For this review, take the finished solid that the model builds, in its own axes (mm). A direction names the side the tool comes from. Coordinates: 2 decimals unless noted, no trailing zeros. Loops run counter-clockwise (first coordinate to the right, second up) from the corner with the lowest first, then second, coordinate; pieces in that order, holes last. Notation, with made-up numbers: (12, 9) - (38, 9) arc R34 cw to (38, 43) - close; hole circle Ø9 at (21.5, 66.25). An arc over 180 degrees is marked (long way). Answer as a JSON object with one key per item and string values. Group by question number.
Item 1: To check wall thickness, follow line 1 (Y direction, x = -9.5, z = 2.2); line 2 (X direction, y = 2, z = 0.35); line 3 (Z direction, x = -26, y = -3). State the ranges of each line that lie inside material, in increasing order.
Item 2: We need section B-B (x = 29). Give the boundary of the cut face in (y, z).
Item 3: We need section A-A (y = 0). State how many separate pieces and enclosed holes the cut face has, then the cut area to 3 significant figures.
Item 4: Mouldability with a two-part tool opening along Y and no side actions: class faces 3 (the flat face through (-50, 0, -0.625)), 4 (the cylindrical face through (-46.01, 14.79, 1.23)), 5 (the cylindrical face through (-45.281, -13.774, 1.866)) as released by +Y, released by -Y, zero draft, split by the parting line, or undercut.
Item 5: Clearance check with flat-ended pins moving along their axes: pin 1 (2 mm diameter, centred on x = 12.5, y = -5, fed in from +Z); pin 2 (6 mm diameter, centred on x = 47, y = 0, fed in from +Z) (3 decimals). State where each tip first meets the part, or that it passes through.
Item 6: Tool access review of faces 1 (the flat face through (-1, 0, 1.25)), 2 (the flat face through (-56, 0, 1)): name each direction out of +Z, -Z, +X, -X, +Y, -Y from which nothing blocks a thin tool from reaching the whole face with its end or side.
from build123d import *

# Parameters (mm, degrees)
BOSS_EXTRUDE1_DEPTH      = 2.5
SKETCH1_3_R              = 3.75
BOSS_EXTRUDE2_DEPTH      = 1.25
BOSS_EXTRUDE4_DEPTH      = 1.875
BOSS_EXTRUDE4_DEPTH_BACK = 0.625
SKETCH1_4_R              = 3.75
SKETCH1_4_R_2            = 2.5


with BuildPart() as part:
    # Sketch1 → Boss-Extrude1 (new body)
    with BuildSketch(Plane.XY):
        with BuildLine():
            ThreePointArc((-53.352941176, 6.898076983), (-55.26649875, 5.541774365), (-56, 3.313942393))
            Line((-56, 3.313942393), (-56, -3.313942393))
            ThreePointArc((-56, -3.313942393), (-55.26649875, -5.541774365), (-53.352941176, -6.898076983))
            ThreePointArc((-53.352941176, -6.898076983), (-49.636038969, -9.136038969), (-47.398076983, -12.852941176))
            ThreePointArc((-47.398076983, -12.852941176), (-46.041774365, -14.76649875), (-43.813942393, -15.5))
            Line((-43.813942393, -15.5), (0, -15.5))
            Line((0, -15.5), (43.813942393, -15.5))
            ThreePointArc((43.813942393, -15.5), (46.041774365, -14.76649875), (47.398076983, -12.852941176))
            ThreePointArc((47.398076983, -12.852941176), (49.636038969, -9.136038969), (53.352941176, -6.898076983))
            ThreePointArc((53.352941176, -6.898076983), (55.26649875, -5.541774365), (56, -3.313942393))
            Line((56, -3.313942393), (56, 3.313942393))
            ThreePointArc((56, 3.313942393), (55.26649875, 5.541774365), (53.352941176, 6.898076983))
            ThreePointArc((53.352941176, 6.898076983), (49.636038969, 9.136038969), (47.398076983, 12.852941176))
            ThreePointArc((47.398076983, 12.852941176), (46.041774365, 14.76649875), (43.813942393, 15.5))
            Line((43.813942393, 15.5), (0, 15.5))
            Line((0, 15.5), (-43.813942393, 15.5))
            ThreePointArc((-43.813942393, 15.5), (-46.041774365, 14.76649875), (-47.398076983, 12.852941176))
            ThreePointArc((-47.398076983, 12.852941176), (-49.636038969, 9.136038969), (-53.352941176, 6.898076983))
        make_face()
        with BuildLine():
            Line((43.813942393, -14.25), (0, -14.25))
            Line((0, -14.25), (-43.813942393, -14.25))
            ThreePointArc((-43.813942393, -14.25), (-45.299163708, -13.760999166), (-46.203365453, -12.485294118))
            ThreePointArc((-46.203365453, -12.485294118), (-48.752155493, -8.252155493), (-52.985294118, -5.703365453))
            ThreePointArc((-52.985294118, -5.703365453), (-54.260999166, -4.799163708), (-54.75, -3.313942393))
            Line((-54.75, -3.313942393), (-54.75, 3.313942393))
            ThreePointArc((-54.75, 3.313942393), (-54.260999166, 4.799163708), (-52.985294118, 5.703365453))
            ThreePointArc((-52.985294118, 5.703365453), (-48.752155493, 8.252155493), (-46.203365453, 12.485294118))
            ThreePointArc((-46.203365453, 12.485294118), (-45.299163708, 13.760999166), (-43.813942393, 14.25))
            Line((-43.813942393, 14.25), (0, 14.25))
            Line((0, 14.25), (43.813942393, 14.25))
            ThreePointArc((43.813942393, 14.25), (45.299163708, 13.760999166), (46.203365453, 12.485294118))
            ThreePointArc((46.203365453, 12.485294118), (48.752155493, 8.252155493), (52.985294118, 5.703365453))
            ThreePointArc((52.985294118, 5.703365453), (54.260999166, 4.799163708), (54.75, 3.313942393))
            Line((54.75, 3.313942393), (54.75, -3.313942393))
            ThreePointArc((54.75, -3.313942393), (54.260999166, -4.799163708), (52.985294118, -5.703365453))
            ThreePointArc((52.985294118, -5.703365453), (48.752155493, -8.252155493), (46.203365453, -12.485294118))
            ThreePointArc((46.203365453, -12.485294118), (45.299163708, -13.760999166), (43.813942393, -14.25))
        make_face(mode=Mode.SUBTRACT)
    extrude(amount=BOSS_EXTRUDE1_DEPTH)

    # Sketch1<3> → Boss-Extrude2 (add)
    with BuildSketch(Plane.XY):
        with BuildLine():
            Line((-43.813942393, -14.25), (0, -14.25))
            Line((0, -14.25), (43.813942393, -14.25))
            ThreePointArc((43.813942393, -14.25), (45.299163708, -13.760999166), (46.203365453, -12.485294118))
            ThreePointArc((46.203365453, -12.485294118), (48.752155493, -8.252155493), (52.985294118, -5.703365453))
            ThreePointArc((52.985294118, -5.703365453), (54.260999166, -4.799163708), (54.75, -3.313942393))
            Line((54.75, -3.313942393), (54.75, 3.313942393))
            ThreePointArc((54.75, 3.313942393), (54.260999166, 4.799163708), (52.985294118, 5.703365453))
            ThreePointArc((52.985294118, 5.703365453), (48.752155493, 8.252155493), (46.203365453, 12.485294118))
            ThreePointArc((46.203365453, 12.485294118), (45.299163708, 13.760999166), (43.813942393, 14.25))
            Line((43.813942393, 14.25), (0, 14.25))
            Line((0, 14.25), (-43.813942393, 14.25))
            ThreePointArc((-43.813942393, 14.25), (-45.299163708, 13.760999166), (-46.203365453, 12.485294118))
            ThreePointArc((-46.203365453, 12.485294118), (-48.752155493, 8.252155493), (-52.985294118, 5.703365453))
            ThreePointArc((-52.985294118, 5.703365453), (-54.260999166, 4.799163708), (-54.75, 3.313942393))
            Line((-54.75, 3.313942393), (-54.75, -3.313942393))
            ThreePointArc((-54.75, -3.313942393), (-54.260999166, -4.799163708), (-52.985294118, -5.703365453))
            ThreePointArc((-52.985294118, -5.703365453), (-48.752155493, -8.252155493), (-46.203365453, -12.485294118))
            ThreePointArc((-46.203365453, -12.485294118), (-45.299163708, -13.760999166), (-43.813942393, -14.25))
        make_face()
        with Locations((-47, 0)):
            Circle(SKETCH1_3_R, mode=Mode.SUBTRACT)
        with Locations((47, 0)):
            Circle(SKETCH1_3_R, mode=Mode.SUBTRACT)
    extrude(amount=BOSS_EXTRUDE2_DEPTH)

    # Sketch1<4> → Boss-Extrude4 (add, two sides: drawn at the far end of the back side and taken through both)
    # profile 1 of 2: a face of its own
    with BuildSketch(Plane.XY.offset(-BOSS_EXTRUDE4_DEPTH_BACK)):
        with Locations((-47, 0)):
            Circle(SKETCH1_4_R)
        with Locations((-47, 0)):
            Circle(SKETCH1_4_R_2, mode=Mode.SUBTRACT)
    # profile 2 of 2: a face of its own
    with BuildSketch(Plane.XY.offset(-BOSS_EXTRUDE4_DEPTH_BACK)):
        with Locations((47, 0)):
            Circle(SKETCH1_4_R)
        with Locations((47, 0)):
            Circle(SKETCH1_4_R_2, mode=Mode.SUBTRACT)
    extrude(amount=BOSS_EXTRUDE4_DEPTH + BOSS_EXTRUDE4_DEPTH_BACK)


solid = part.part
Check sheet entries:
{
 "1": {"line 1": "y = -15.5 to -14.25, 14.25 to 15.5", "line 2": "x = -56 to -48.5, -45.5 to 45.5, 48.5 to 56", "line 3": "z = 0 to 1.25"},
 "2": {"outline": "(-15.5, 0) - (15.5, 0) - (15.5, 2.5) - (14.25, 2.5) - (14.25, 1.25) - (-14.25, 1.25) - (-14.25, 2.5) - (-15.5, 2.5) - close"},
 "3": {"separate pieces": "3", "enclosed holes": "0", "area": "137 mm2"},
 "4": {"face 3": "zero draft", "face 4": "released by +Y", "face 5": "undercut"},
 "5": {"pin 1": "stops at z = 1.25", "pin 2": "stops at z = 1.875"},
 "6": {"face 1": "+Z", "face 2": "+Z, -Z, -X, +Y, -Y"}
}
